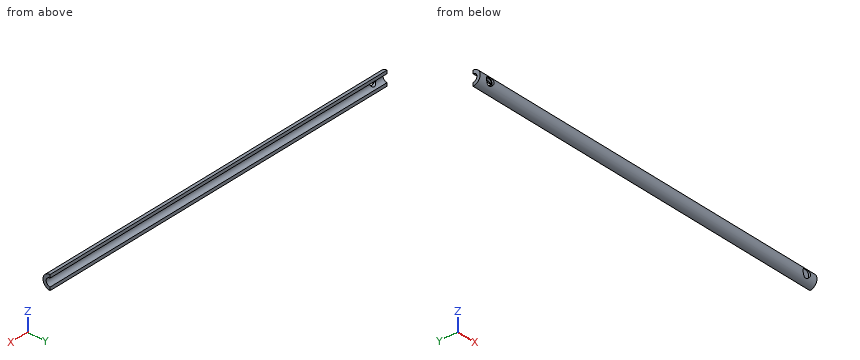
```python
from build123d import *

# Parameters (mm, degrees)
SKETCH1_W                     = 735.584
SKETCH1_H                     = 38.1
WOOD_BLOCK_DEPTH              = 15.875
SKETCH2_R                     = 7.9375
INNER_BORE_DEPTH              = 737.741098814
SKETCH3_R                     = 6.35
MOUTHPIECE_THROUGH_HOLE_DEPTH = 737.741098814
SKETCH5_R                     = 8.128
CUT_EXTRUDE3_DEPTH            = 5.5499
SKETCH6_R                     = 8.128
CUT_EXTRUDE4_DEPTH            = 5.3975
SKETCH4_OUTSIDE_W             = 187.448
SKETCH4_OUTSIDE_H             = 165.223
SKETCH4_OUTSIDE_R             = 14.2875
OUTER_DIAMETER_DEPTH          = 737.741098916


with BuildPart() as part:
    # Sketch1 → wood block (new body)
    with BuildSketch(Plane(origin=(0, 0, 0), x_dir=(1, 0, 0), z_dir=(0, 1, 0))):
        with Locations((367.792, 19.05)):
            Rectangle(SKETCH1_W, SKETCH1_H)
    extrude(amount=WOOD_BLOCK_DEPTH)

    # Sketch2 → inner bore (cut, through all)
    with BuildSketch(Plane(origin=(735.584, 0, 0), x_dir=(0, 0, -1), z_dir=(1, 0, 0))):
        with Locations((19.05, 15.875)):
            Circle(SKETCH2_R)
    extrude(amount=-INNER_BORE_DEPTH, mode=Mode.SUBTRACT)

    # Sketch3 → mouthpiece through hole (cut, through all)
    with BuildSketch(Plane(origin=(0, 0, 0), x_dir=(1, 0, 0), z_dir=(0, 1, 0))):
        with Locations(Location((22.225, 19.05, 0), (0, 0, 90))):
            Circle(SKETCH3_R)
    extrude(amount=MOUTHPIECE_THROUGH_HOLE_DEPTH, mode=Mode.SUBTRACT)

    # Sketch5 → Cut-Extrude3 (cut)
    with BuildSketch(Plane.XZ):
        with Locations(Location((22.225, -19.05, 0), (0, 0, 270))):
            Circle(SKETCH5_R)
    extrude(amount=-CUT_EXTRUDE3_DEPTH, mode=Mode.SUBTRACT)

    # Sketch6 → Cut-Extrude4 (cut)
    with BuildSketch(Plane.XZ):
        with Locations(Location((713.359, -19.05, 0), (0, 0, 270))):
            Circle(SKETCH6_R)
    extrude(amount=-CUT_EXTRUDE4_DEPTH, mode=Mode.SUBTRACT)

    # Sketch4 outside → outer diameter (cut, through all)
    with BuildSketch(Plane.ZY):
        with Locations((-19.05, 7.9375)):
            Rectangle(SKETCH4_OUTSIDE_W, SKETCH4_OUTSIDE_H)
        with Locations((-19.05, 15.875)):
            Circle(SKETCH4_OUTSIDE_R, mode=Mode.SUBTRACT)
    extrude(amount=-OUTER_DIAMETER_DEPTH, mode=Mode.SUBTRACT)


solid = part.part
```
Work out the finished part from the listing and answer in its coordinate system (mm). Give positions to 0.01 mm unless a question says otherwise; leave off trailing zeros. Loops run counter-clockwise (first coordinate to the right, second up) from the corner with the lowest first, then second, coordinate; pieces in that order, holes last. Notation, with made-up numbers: M -24,-15 L 11,-15 A17 cw 11,10 Z; hole C 33,43.5 d3. An arc over 180 degrees is marked long. One line per item, written item: value. Start each with the question number.
1. Find the intervals of material crossed by probe 1 along X at (y, z) = (2.55, -19.05); probe 2 along Z at (x, y) = (252, 14.5); probe 3 along Y at (x, z) = (180.5, -29) (3 decimals), in increasing order.
2. Each of these flat-tipped pins is pushed along its axis until it touches: P1, Ø4, axis at x = 156, y = 5.5, coming from the +Z side; P2, Ø4, axis at x = 626.5, z = -14, coming from the +Y side; P3, Ø1, axis at x = 161, y = 5.5, coming from the +Z side. Where does it stop, or does it pass through?
3. Find section A-A (z = -19.05). Give the vertices of the cut face in (x, y) (1 decimal).
Reported:
1. probe 1: x = 0 to 14.1, 30.35 to 705.23, 721.49 to 735.58
1. probe 2: z = -33.27 to -26.87, -11.23 to -4.83
1. probe 3: y = 5.622 to 15.875
2. P1: stops at z = -7.47
2. P2: stops at y = 12.23
2. P3: stops at z = -8.72
3. outline: M 0,1.6 L 14.1,1.6 L 14.1,5.5 L 15.9,5.5 L 15.9,7.9 L 0,7.9 Z; M 28.6,5.5 L 30.4,5.5 L 30.4,1.6 L 705.2,1.6 L 705.2,5.4 L 721.5,5.4 L 721.5,1.6 L 735.6,1.6 L 735.6,7.9 L 28.6,7.9 Z
